```python
from build123d import *

# Parameters (mm, degrees)
SKETCH1_R           = 60
BOSS_EXTRUDE1_DEPTH = 5.08
SKETCH2_R           = 2.1828125
CUT_EXTRUDE1_DEPTH  = 6.08
CIRPATTERN1_COUNT   = 2
CIRPATTERN1_ANGLE   = 120
SKETCH3_R           = 1.5
CUT_EXTRUDE2_DEPTH  = 6.08
SKETCH5_R           = 2.1828125
CUT_EXTRUDE4_DEPTH  = 6.08
SKETCH6_R           = 19.05
CUT_EXTRUDE5_DEPTH  = 6.08
SKETCH9_W           = 17
SKETCH9_H           = 13
BOSS_EXTRUDE2_DEPTH = 5.08
SKETCH7_R           = 1.5
CUT_EXTRUDE6_DEPTH  = 6.08
FILLET1_R           = 2
FILLET2_R           = 2


with BuildPart() as part:
    # Sketch1 → Boss-Extrude1 (new body)
    with BuildSketch(Plane(origin=(0, 0, 0), x_dir=(1, 0, 0), z_dir=(0, 1, 0))):
        Circle(SKETCH1_R)
    extrude(amount=BOSS_EXTRUDE1_DEPTH)

    # Sketch2 → Cut-Extrude1 (cut, through all)
    with BuildSketch(Plane(origin=(0, 5.08, 0), x_dir=(1, 0, 0), z_dir=(0, 1, 0))):
        with Locations((-36.386057378, -21.007500022)):
            Circle(SKETCH2_R)
    cut_extrude1 = extrude(amount=-CUT_EXTRUDE1_DEPTH, mode=Mode.SUBTRACT)

    # CirPattern1: Cut-Extrude1 ×2 about axis
    cirpattern1_axis = Axis((0, 5.08, 0), (0, 1, 0))
    for i in range(1, CIRPATTERN1_COUNT):
        add(cut_extrude1.rotate(cirpattern1_axis, i * CIRPATTERN1_ANGLE / (CIRPATTERN1_COUNT - 1)), mode=Mode.SUBTRACT)

    # Sketch3 → Cut-Extrude2 (cut, through all)
    with BuildSketch(Plane(origin=(0, 5.08, 0), x_dir=(1, 0, 0), z_dir=(0, 1, 0))):
        with Locations((-6.5, 6.749999962)):
            Circle(SKETCH3_R)
        with Locations((6.5, 6.749999962)):
            Circle(SKETCH3_R)
        with Locations((-12.5, 33.500000056)):
            Circle(SKETCH3_R)
        with Locations((12.5, 33.500000056)):
            Circle(SKETCH3_R)
        with Locations((35.421216966, 27.378652381)):
            Circle(SKETCH3_R)
        with Locations((41.421216966, 16.986347535)):
            Circle(SKETCH3_R)
        with Locations((-45.294385987, 18.067822174)):
            Circle(SKETCH3_R)
        with Locations((-38.294385987, 30.192177826)):
            Circle(SKETCH3_R)
    extrude(amount=-CUT_EXTRUDE2_DEPTH, mode=Mode.SUBTRACT)

    # Sketch5 → Cut-Extrude4 (cut, through all)
    with BuildSketch(Plane(origin=(0, 5.08, 0), x_dir=(1, 0, 0), z_dir=(0, 1, 0))):
        with Locations((-22.5, 25)):
            Circle(SKETCH5_R)
        with Locations((22.5, 25)):
            Circle(SKETCH5_R)
    extrude(amount=-CUT_EXTRUDE4_DEPTH, mode=Mode.SUBTRACT)

    # Sketch6 → Cut-Extrude5 (cut, through all)
    with BuildSketch(Plane(origin=(0, 5.08, 0), x_dir=(1, 0, 0), z_dir=(0, 1, 0))):
        with Locations((0, -25.4)):
            Circle(SKETCH6_R)
    extrude(amount=-CUT_EXTRUDE5_DEPTH, mode=Mode.SUBTRACT)

    # Sketch9 → Boss-Extrude2 (add)
    with BuildSketch(Plane(origin=(0, 5.08, 0), x_dir=(1, 0, 0), z_dir=(0, 1, 0))):
        with Locations((0, -65.894865098)):
            Rectangle(SKETCH9_W, SKETCH9_H)
    extrude(amount=-BOSS_EXTRUDE2_DEPTH)

    # Sketch7 → Cut-Extrude6 (cut, through all)
    with BuildSketch(Plane(origin=(0, 5.08, 0), x_dir=(1, 0, 0), z_dir=(0, 1, 0))):
        with Locations((-9, -47)):
            Circle(SKETCH7_R)
        with Locations((-6, -67.394865098)):
            Circle(SKETCH7_R)
        with Locations((6, -67.394865098)):
            Circle(SKETCH7_R)
        with Locations((9, -47)):
            Circle(SKETCH7_R)
        with BuildLine():
            Line((-4.445, -60.964865098), (-4.445, -43.924159225))
            Line((-4.445, -43.924159225), (4.445, -43.924159225))
            Line((4.445, -43.924159225), (4.445, -60.964865098))
            ThreePointArc((4.445, -60.964865098), (0, -65.409865098), (-4.445, -60.964865098))
        make_face()
    extrude(amount=-CUT_EXTRUDE6_DEPTH, mode=Mode.SUBTRACT)

    # Fillet1
    fillet1_edges = [part.edges().sort_by_distance(p)[0] for p in [
        (8.5, 2.54, 72.394865098),
        (-8.5, 2.54, 72.394865098),
    ]]
    fillet(fillet1_edges, radius=FILLET1_R)

    # Fillet2
    fillet2_edges = [part.edges().sort_by_distance(p)[0] for p in [
        (8.5, 2.54, 59.394865098),
        (-8.5, 2.54, 59.394865098),
    ]]
    fillet(fillet2_edges, radius=FILLET2_R)


solid = part.part
```
Check sheet for the modelled part. Datum: model origin and axes. Units: mm. A direction names the side the tool comes from. Round coordinates to 2 decimals unless told otherwise and drop trailing zeros. Order: outer loops, then holes, each group sorted by start corner. A loop starts at its lowest first (then second) coordinate and runs counter-clockwise, first axis right, second up. Notation, with made-up numbers: (70.25, 34.25) - (117.25, 34.25) arc R18 cw to (117.25, 59.25) - close; hole circle Ø7 at (70, 22.25). An arc over 180 degrees is marked (long way). Answer as CSV lines item,"result". Start each with the question number.
1) Section check B-B (z = 47). Record the cut outline in (x, y) (3 decimals).
2) Tool access check on faces 4 (the face through (8.5, 3, 66)), 5 (the face through (0.1, 2.58, 65.41)), 6 (the face through (-1, 5.08, -9)). Record the directions out of +Z, -Z, +X, -X, +Y, -Y that give a thin tool (end or side, any length) a straight path to the whole face; none if there is none.
3) Section check C-C (y = 2.7). Give the number of separate pieces and of enclosed holes in the cut face, then the cut area to 3 significant figures.
4) Section check D-D (x = -22.5). Record the cut outline in (y, z), then the cut area to 3 significant figures.
5) Draft check along X on faces 1 (the face through (2.495, 2.504, -59.948)), 2 (the face through (-7.61, 2.58, -7.76)), 3 (the face through (-1, 0, -9)). Enter one of: +X half, -X half, draft (parallel to the pull), parting line (faces both ways), or undercut.
6) Depth check by flat-ended pin: pin 1 (1.5 mm diameter, centred on y = 2.5, z = 65, fed in from -X); pin 2 (2 mm diameter, centred on x = -18, y = 4, fed in from -Z). Enter the tip coordinate at first touch or a pass-through.
7) Scan lines: probe 1 along X at (y, z) = (2.4, 47) (3 decimals); probe 2 along Z at (x, y) = (12, 0.9); probe 3 along Z at (x, y) = (-12.5, 1.85). Record each from-to range of solid material in increasing order.
8) Section check A-A (x = 12.5). Record the cut outline in (y, z).
Determined:
1,outline,"(-37.296, 0) - (-10.5, 0) - (-10.5, 5.08) - (-37.296, 5.08) - close; (-7.5, 0) - (-4.445, 0) - (-4.445, 5.08) - (-7.5, 5.08) - close; (4.445, 0) - (7.5, 0) - (7.5, 5.08) - (4.445, 5.08) - close; (10.5, 0) - (37.296, 0) - (37.296, 5.08) - (10.5, 5.08) - close"
2,face 4,"+Z, +X, +Y, -Y"
2,face 5,"+Y, -Y"
2,face 6,"+Z, -Z, +X, -X, +Y"
3,separate pieces,"1"
3,enclosed holes,"17"
3,area,"10,100 mm^2"
4,outline,"(0, -55.62) - (5.08, -55.62) - (5.08, -27.18) - (0, -27.18) - close; (0, -22.82) - (5.08, -22.82) - (5.08, 55.62) - (0, 55.62) - close"
4,area,"543 mm^2"
5,face 1,"parting line"
5,face 2,"undercut"
5,face 3,"draft"
6,pin 1,"x = -8.5"
6,pin 2,"z = -57.54"
7,probe 1,"-37.296 to -10.5, -7.5 to -4.445, 4.445 to 7.5, 10.5 to 37.296"
7,probe 2,"-58.79 to -34.91, -32.09 to 10.6, 40.2 to 58.79"
7,probe 3,"-58.68 to -35, -32 to 11.02, 39.78 to 58.68"
8,outline,"(0, -58.68) - (5.08, -58.68) - (5.08, -35) - (0, -35) - close; (0, -32) - (5.08, -32) - (5.08, 11.02) - (0, 11.02) - close; (0, 39.78) - (5.08, 39.78) - (5.08, 58.68) - (0, 58.68) - close"
